```python
from build123d import *

# Parameters (mm, degrees)
SKETCH_2_W          = 280
SKETCH_2_H          = 150
EXTRUDE_1_DEPTH     = 5
SKETCH_3_W          = 280
SKETCH_3_H          = 25
EXTRUDE_2_DEPTH     = 10
CUT_EXTRUDE_1_DEPTH = 25
SKETCH_5_R          = 4
CUT_EXTRUDE_2_DEPTH = 50
SKETCH_6_W          = 5
SKETCH_6_H          = 160
EXTRUDE_3_DEPTH     = 20
EXTRUDE_4_DEPTH     = 5
CUT_EXTRUDE_3_DEPTH = 20
SKETCH_9_W          = 112.05
SKETCH_9_H          = 25
CUT_EXTRUDE_4_DEPTH = 20
FILLET_1_R          = 2


with BuildPart() as part:
    # 草图2 → 凸台-拉伸1 (new body)
    with BuildSketch(Plane.XY):
        Rectangle(SKETCH_2_W, SKETCH_2_H)
    extrude(amount=EXTRUDE_1_DEPTH)

    # 草图3 → 凸台-拉伸2 (add)
    with BuildSketch(Plane(origin=(0, 75, 0), x_dir=(1, 0, 0), z_dir=(0, 1, 0))):
        with Locations((0, 12.5)):
            Rectangle(SKETCH_3_W, SKETCH_3_H)
    extrude(amount=-EXTRUDE_2_DEPTH)

    # 草图4 → 切除-拉伸1 (cut, symmetric)
    with BuildSketch(Plane(origin=(0, 0, 0), x_dir=(-1, 0, 0), z_dir=(0, 0, -1))):
        Polygon((75.462063134, 103.147200408), (-172.007852349, -104.504714401), (179.32828037, -108.521449105), (159.998225544, 98.6463124), align=None)
    extrude(amount=CUT_EXTRUDE_1_DEPTH, both=True, mode=Mode.SUBTRACT)

    # 草图5 → 切除-拉伸2 (cut)
    with BuildSketch(Plane.XZ.offset(-65)):
        with Locations(Location((-20, -15, 0), (0, 0, 270))):
            Circle(SKETCH_5_R)
        with Locations(Location((10, -15, 0), (0, 0, 270))):
            Circle(SKETCH_5_R)
    extrude(amount=-CUT_EXTRUDE_2_DEPTH, mode=Mode.SUBTRACT)

    # 草图6 → 凸台-拉伸3 (add)
    with BuildSketch(Plane(origin=(140, 0, 0), x_dir=(0, 0, -1), z_dir=(1, 0, 0))):
        with Locations((-2.5, -5)):
            Rectangle(SKETCH_6_W, SKETCH_6_H)
    extrude(amount=EXTRUDE_3_DEPTH)

    # 草图7 → 凸台-拉伸4 (add)
    with BuildSketch(Plane.XY.offset(5)):
        Polygon((136.845502963, -75), (140, -77.6469373), (140, -75), align=None)
    extrude(amount=-EXTRUDE_4_DEPTH)

    # 草图8 → 切除-拉伸3 (cut)
    with BuildSketch(Plane.XY.offset(5)):
        Polygon((140, -77.6469373), (153.856787924, -89.274162936), (129.719459365, -89.898808536), align=None)
    extrude(amount=-CUT_EXTRUDE_3_DEPTH, mode=Mode.SUBTRACT)

    # 草图9 → 切除-拉伸4 (cut)
    with BuildSketch(Plane.XZ.offset(-65)):
        with Locations((83.975, -12.5)):
            Rectangle(SKETCH_9_W, SKETCH_9_H)
    extrude(amount=-CUT_EXTRUDE_4_DEPTH, mode=Mode.SUBTRACT)

    # 圆角1
    fillet_1_edges = [part.edges().sort_by_distance(p)[0] for p in [
        (27.95, 70, 0),
        (-1.025, 65, 0),
    ]]
    fillet(fillet_1_edges, radius=FILLET_1_R)


solid = part.part
```
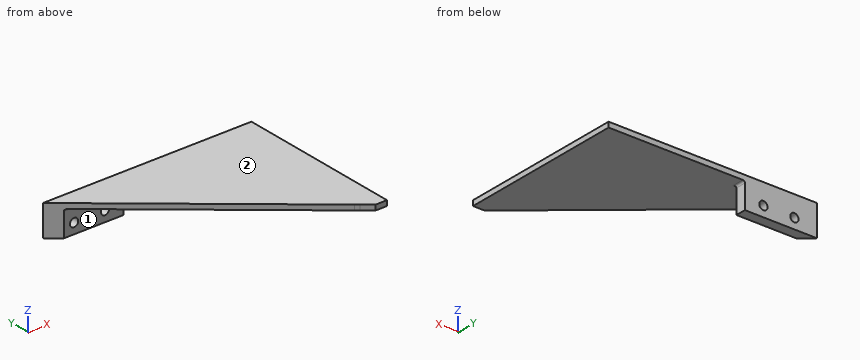
The listing builds one solid part. Answer for the finished solid, in the listing's coordinates (mm). Face numbers are marked on the shaded views. A direction names the side the tool comes from. Round coordinates to 2 decimals unless told otherwise and drop trailing zeros. Loops run counter-clockwise (first coordinate to the right, second up) from the corner with the lowest first, then second, coordinate; pieces in that order, holes last. Notation, with made-up numbers: (24.25, 36) - (32.25, 36) arc R18 cw to (32.25, 49) - close; hole circle Ø8 at (14.25, 9.5). An arc over 180 degrees is marked (long way). Return JSON: item names as keys, results as strings. Group by question number.
1. The part is cut by section C-C on x = 17.5. Determine the outline of the cut face in (y, z).
2. Consider probe 1 along X at (y, z) = (71.5, -15); probe 2 along Z at (x, y) = (147, 20); probe 3 along X at (y, z) = (41.5, 0.5). Determine where each line is inside the solid, lowest interval first.
3. The part is cut by section B-B on x = -20. Determine the outline of the cut face in (y, z), then the cut area to 3 significant figures.
4. Which of the six approach directions +Z, -Z, +X, -X, +Y, -Y give full straight-line access (tool end or side, diameter ignored) to the marked faces 1 and 2?
5. Each of these flat-tipped pins is pushed along its axis until it touches: P1, Ø10.5, axis at x = -20, z = -15, coming from the -Y side; P2, Ø3, axis at y = 70, z = -8, coming from the +X side. Where does it stop, or does it pass through?
6. The part is cut by section A-A on z = -15. Determine the outline of the cut face in (x, y), then the cut area to 3 significant figures.
7. The part is cut by section D-D on y = 12. Determine the outline of the cut face in (x, z).
Resolved:
{
 "1": {"outline": "(25.14, 0) - (63, 0) arc R2 cw to (65, -2) - (65, -25) - (75, -25) - (75, 5) - (25.14, 5) - close"},
 "2": {"probe 1": "x = -37.75 to -24, -16 to 6, 14 to 27.95", "probe 2": "z = 0 to 5", "probe 3": "x = -1.99 to 160"},
 "3": {"outline": "(56.61, 0) - (63, 0) arc R2 cw to (65, -2) - (65, -11) - (75, -11) - (75, 5) - (56.61, 5) - close; (65, -25) - (75, -25) - (75, -19) - (65, -19) - close", "area": "263 mm²"},
 "4": {"face 1": "-Z, +X, -X, -Y", "face 2": "+Z, +X, -X, +Y, -Y"},
 "5": {"P1": "stops at y = 65", "P2": "stops at x = 27.95"},
 "6": {"outline": "(-41.92, 75) - (-30, 65) - (-24, 65) - (-24, 75) - close; (-16, 65) - (6, 65) - (6, 75) - (-16, 75) - close; (14, 65) - (27.95, 65) - (27.95, 75) - (14, 75) - close", "area": "479 mm²"},
 "7": {"outline": "(33.16, 0) - (160, 0) - (160, 5) - (33.16, 5) - close"}
}
